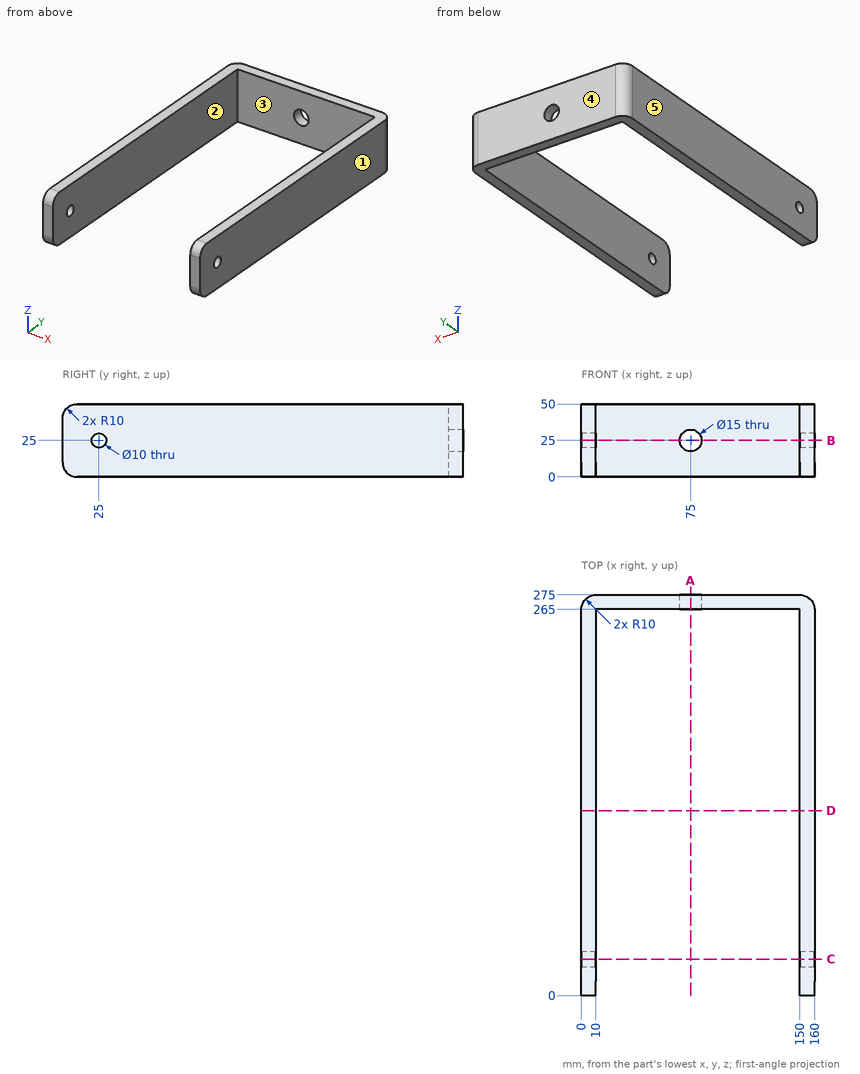
Print and shaded views of the part. All mm, measured from the part's lowest x, y and z. A direction names the side the tool comes from. Coordinates: 2 decimals unless noted, no trailing zeros. Write each loop counter-clockwise with the first axis right and the second up, starting at its lowest first coordinate (ties: lowest second). Pieces come first, ordered by that corner, then holes.
(1) Cut at A-A, the plane x = 75. List the corners of the cut face in (y, z), and give its area (3 significant figures).
(2) Cut at B-B, the plane z = 25. List the corners of the cut face in (x, y).
(3) Cut at C-C, the plane y = 25. List the corners of the cut face in (x, z).
(4) Flat gauge pins, fed straight in: pin 1 (1 mm diameter, centred on x = 137, z = 14, fed in from -Y); pin 2 (9 mm diameter, centred on x = 75, z = 25, fed in from +Y). Where does each tip first touch, or does it go through?
(5) Two-plate mould, pull along X, no slides. Class the marked faces 3, 4 and 5: +X half, -X half, draft (parallel to the pull), parting line (faces both ways), or undercut.
(6) Drill centre lines: probe 1 along X at (y, z) = (146, 11.5); probe 2 along Z at (x, y) = (4.25, 25); probe 3 along Y at (x, z) = (73.5, 37). Where is each one in solid material? Low to high.
(7) 3-axis set-ups, long thin cutter, end or side, ignore diameter. For the marked faces 1 and 2: which of +Z, -Z, +X, -X, +Y, -Y reach the whole face in a straight line?
(8) Cut at D-D, the plane y = 127. List the corners of the cut face in (x, z).
Geometry says:
1. outline: (265, 0) - (275, 0) - (275, 17.5) - (265, 17.5) - close; (265, 32.5) - (275, 32.5) - (275, 50) - (265, 50) - close
1. area: 350 mm2
2. outline: (0, 0) - (10, 0) - (10, 20) - (0, 20) - close; (0, 30) - (10, 30) - (10, 265) - (67.5, 265) - (67.5, 275) - (10, 275) arc R10 ccw to (0, 265) - close; (82.5, 265) - (150, 265) - (150, 30) - (160, 30) - (160, 265) arc R10 ccw to (150, 275) - (82.5, 275) - close; (150, 0) - (160, 0) - (160, 20) - (150, 20) - close
3. outline: (0, 0) - (10, 0) - (10, 20) - (0, 20) - close; (0, 30) - (10, 30) - (10, 50) - (0, 50) - close; (150, 0) - (160, 0) - (160, 20) - (150, 20) - close; (150, 30) - (160, 30) - (160, 50) - (150, 50) - close
4. pin 1: stops at y = 265
4. pin 2: passes through
5. face 3: undercut
5. face 4: draft
5. face 5: -X half
6. probe 1: x = 0 to 10, 150 to 160
6. probe 2: z = 0 to 20, 30 to 50
6. probe 3: y = 265 to 275
7. face 1: +Z, -Z, +X, +Y, -Y
7. face 2: +Z, -Z, -Y
8. outline: (0, 0) - (10, 0) - (10, 50) - (0, 50) - close; (150, 0) - (160, 0) - (160, 50) - (150, 50) - close
